```python
from build123d import *

# Parameters (mm, degrees)
F2_R = 2.61643


with BuildPart() as f1:
    # F0 (on Top) → F1 (revolve)
    with BuildSketch(Plane.XY):
        Polygon((-55.398632, 0), (0, 0), (0, 38.622338), (-13.734436, 20.002501), (-16.695562, 20.177716), (-44.890404, 21.84605), (-55.398632, 38.622338), align=None)
    revolve(axis=Axis((0, 19.311169, 0), (0, 1, 0)))

    # F2
    f2_edges = [f1.edges().sort_by_distance(p)[0] for p in [
        (55.398632, 38.622338, 0),
    ]]
    fillet(f2_edges, radius=F2_R)


solid = f1.part
```
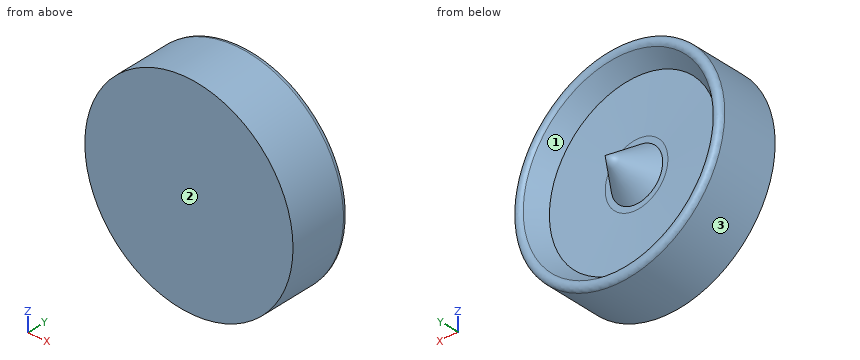
The model under review builds one solid part; all positions refer to its coordinate system, in mm. Face numbers are marked on the shaded views. Coordinates: 2 decimals unless noted, no trailing zeros. Order: outer loops, then holes, each group sorted by start corner. A loop starts at its lowest first (then second) coordinate and runs counter-clockwise, first axis right, second up. Notation, with made-up numbers: M 5,-22.75 L 10,-22.75 A12 ccw 10,-1.75 Z; hole C -10,-23 d4. An arc over 180 degrees is marked long. One line per question, with ' | ' between items.
(1) Insertion check: pin 1 (5 mm diameter, centred on x = -42, y = 17.5, fed in from +Z); pin 2 (12 mm diameter, centred on y = 21, z = -8.5, fed in from +X); pin 3 (3 mm diameter, centred on x = 31.5, z = -40, fed in from -Y); pin 4 (3 mm diameter, centred on x = -4.5, y = 8.5, fed in from +Z). Each pin has a flat end and moves straight along its axis. Give the tip position at first contact, or say it passes through.
Geometry results:
pin 1: stops at z = 38.84 | pin 2: stops at x = 55.34 | pin 3: stops at y = 0 | pin 4: stops at z = 55.32
(2) Add section A-A, the plane y = 17.5. Write out the cut boundary in (x, z), then the cut area to 3 significant figures.
Geometry results:
outline: C 0,0 d110.8 | area: 9,640 mm²
(3) Add section B-B, the plane y = 35.5. Write out the cut boundary in (x, z), then the cut area to 3 significant figures.
Geometry results:
outline: C 0,0 d4.61 | area: 16.7 mm²
(4) The part is to be moulded in two halves that separate along X. For the marked faces 1, 2 and 3, say which applies: +X half, -X half, draft (parallel to the pull), parting line (faces both ways), or undercut.
Geometry results:
face 1: undercut | face 2: draft | face 3: parting line
(5) For probe 1 along X at (y, z) = (30, 1.5); probe 2 along X at (y, z) = (24.5, -28.5); probe 3 along Z at (x, y) = (10, 23.5), list the stretches that pass through material, from the lowest coordinate up. Write a range as from..to.
Geometry results:
probe 1: x = -55.33..-49.98, -6.18..6.18, 49.98..55.33 | probe 2: x = -47.51..-36.81, 36.81..47.51 | probe 3: z = -54.49..-44.82, -4.94..4.94, 44.82..54.49
